Part model, mm, in its own coordinate system. A direction names the side the tool comes from. Round coordinates to 2 decimals unless told otherwise and drop trailing zeros. Write each loop counter-clockwise with the first axis right and the second up, starting at its lowest first coordinate (ties: lowest second). Pieces come first, ordered by that corner, then holes. Notation, with made-up numbers: M -18,12.25 L -9,12.25 A24 cw -9,46.25 Z; hole C 85,23 d11. An arc over 180 degrees is marked long. Use one line per item in the form item = value. Start each with the question number.
Item 1: Which spindle directions (+Z, -Z, +X, -X, +Y, -Y) get a long thin tool onto all of the face, cutting with end or side? Do faces 1 (the face through (14.45, 18.73, 22.38)), 2 (the face through (9.4, 3.55, -0.57)), 3 (the face through (15.64, 18.43, 23.66)). Say none if no direction does.
Item 2: Flat gauge pins, fed straight in: pin 1 Ø10 at (x, z) = (10, 25.5) entering from -Y; pin 2 Ø11 at (x, z) = (8.5, -6) entering from +Y; pin 3 Ø3 at (x, y) = (4.5, 3) entering from +Z; pin 4 Ø10 at (y, z) = (15.5, 4) entering from +X. Where does each tip first touch, or does it go through?
Item 3: Mould opens along Z. For faces 4 (the face through (6, 10, 2)), 5 (the face through (5, 3, -15)), 6 (the face through (15.94, 10.14, 23.33)) say: +Z half, -Z half, draft (parallel to the pull), parting line (faces both ways), or undercut.
Item 4: Cut at B-B, the plane x = 4. Give the cut face in (y, z).
Item 5: Cut at A-A, the plane y = 3. Give the cut face in (x, z).
Item 6: Cut at D-D, the plane z = -3.5. Give the cut face in (x, y).
Item 7: Probe L1, parallel to Y at x = 7, z = -16.5; L2, parallel to Z at x = 4.75, y = 4; L3, parallel to Y at x = 6, z = -9. List the from-to ranges inside material, lowest first.
Item 8: Cut at C-C, the plane y = 8.25. Give the cut face in (x, z).
Autodesk Inventor part; units mm, degrees
ref_plane "YZ Plane" through (0, 0, 0) normal (1, 0, 0) x (0, 1, 0)
ref_plane "XZ Plane" through (0, 0, 0) normal (0, 1, 0) x (-1, 0, 0)
ref_plane "XY Plane" through (0, 0, 0) normal (0, 0, 1) x (1, 0, 0)
sketch "Náčrt1" plane through (0, 0, 0) normal (0, 1, 0) x (-1, 0, 0)
  line L0 (0, 0) -> (-10, 0)
  line L1 (-10, 0) -> (-10, -5)
  line L2 (-10, -5) -> (0, -5)
  line L3 (0, -5) -> (0, 0)
  line L4 (0, -15) -> (-10, -15)
  line L5 (-10, -15) -> (-10, -20)
  line L6 (-10, -20) -> (0, -20)
  line L7 (0, -20) -> (0, -15)
  dimension "d0" = 10
  dimension "d1" = 5
  dimension "d2" = 5
  dimension "d3" = 10
extrude "Vysunutí1" add sketch "Náčrt1" along normal blind 7
sketch "Náčrt2" plane through (0, 7, 0) normal (0, 1, 0) x (1, 0, 0)
  line L0 (0, 0) -> (10, 0)
  line L1 (10, 0) -> (10, 20)
  line L2 (10, 20) -> (0, 20)
  line L3 (0, 20) -> (0, 0)
  line L4 (10, 0) -> (10, 5)
  line L5 (10, 0) -> (0, 0)
  line L6 (0, 0) -> (0, -10)
  line L7 (0, -10) -> (10, -10)
  line L8 (10, -10) -> (10, 0)
  line L9 (10, -10) -> (25, -25)
  line L10 (0, -10) -> (15, -25)
  line L11 (25, -25) -> (15, -25)
  dimension "d6" = 10
  dimension "d7" = 10
  dimension "d8" = 135
  dimension "d9" = 15
  dimension "d10" = 15
extrude "Vysunutí2" add sketch "Náčrt2" along normal blind 3
sketch "Náčrt3" plane through (0, 10, 0) normal (0, 1, 0) x (1, 0, 0)
  line L0 (15, -25) -> (25, -25)
  line L1 (17.328427, -24.5) -> (14.828427, -22)
  line L2 (14.828427, -22) -> (17.328427, -19.5)
  line L3 (17.328427, -19.5) -> (19.828427, -22)
  line L4 (19.828427, -22) -> (17.328427, -24.5)
  line L5 (0, -10) -> (15, -25)
  point P0 (0, 0)
  dimension "d22" = 2.5
  dimension "d23" = 2.5
  dimension "d24" = 0.5
  dimension "d25" = 2
extrude "Vysunutí5" add sketch "Náčrt3" along normal blind 12
sketch "Náčrt5" plane through (17.328427, 10, 24.5) normal (-0.7071068, 0, 0.7071068) x (0.7071068, 0, 0.7071068)
  line L0 (0, 12) -> (-3.535534, 12)
  line L1 (0, 0) -> (0, 12)
  line L2 (-3.535534, 12) -> (0, 12)
  line L3 (0, 12) -> (0, 9)
  line L4 (0, 9) -> (-3.535534, 9)
  line L5 (-3.535534, 9) -> (-3.535534, 12)
  point P0 (-29.577164, -10)
  dimension "d28" = 3
extrude "Vysunutí6" add sketch "Náčrt5" along normal blind 12
fillet "Zaoblení1" radius 2 8 edges at (25, 8.5, 25) (15, 8.5, 25) (10, 8.5, 10) (0, 8.5, 10) (10, 5, -20) (0, 5, -20) (0, 3.5, 0) (10, 3.5, 0)
fillet "Zaoblení2" radius 2 1 edges at (16.0784, 19, 23.25)
fillet "Zaoblení3" radius 0.5 4 edges at (16.0784, 10, 20.75) (16.0784, 10, 23.25) (18.5784, 10, 20.75) (18.5784, 10, 23.25)
fillet "Zaoblení4" radius 2 1 edges at (18.5784, 22, 20.75)
fillet "Zaoblení5" radius 0.5 4 edges at (7.5931, 22, 31.7353) (7.5931, 19, 31.7353) (8.8431, 20.5, 32.9853) (6.3431, 20.5, 30.4853)
equation "\"d10\" = d9"
properties part number "NozzleCleaner"
Model answer:
q1.face_1 = -Z, -X, +Y
q1.face_2 = +Z, +X, -Y
q1.face_3 = +Z, -X
q2.pin_1 = 7
q2.pin_2 = 10
q2.pin_3 = 0
q2.pin_4 = through
q3.face_4 = draft
q3.face_5 = undercut
q3.face_6 = +Z half
q4.outline = M 0,-20 L 10,-20 L 10,14 L 7,14 L 7,0 L 0,0 L 0,-5 L 7,-5 L 7,-15 L 0,-15 Z
q5.outline = M 0,-18 A2 ccw 2,-20 L 8,-20 A2 ccw 10,-18 L 10,-15 L 0,-15 Z; M 0,-5 L 10,-5 L 10,-2 A2 ccw 8,0 L 2,0 A2 ccw 0,-2 Z
q6.outline = M 0,0 L 10,0 L 10,10 L 0,10 Z
q7.L1 = 0 to 10
q7.L2 = -20 to -15, -5 to 0
q7.L3 = 7 to 10
q8.outline = M 0,-18 A2 ccw 2,-20 L 8,-20 A2 ccw 10,-18 L 10,9.17 A2 cw 10.59,10.59 L 21.59,21.59 A2 ccw 20.17,25 L 15.83,25 A2 ccw 14.41,24.41 L 0.59,10.59 A2 ccw 0,9.17 Z
